Verification items for the finished model (mm, model axes). Round coordinates to 2 decimals unless told otherwise and drop trailing zeros. Order: outer loops, then holes, each group sorted by start corner. A loop starts at its lowest first (then second) coordinate and runs counter-clockwise, first axis right, second up. Notation, with made-up numbers: (73, -32.5) -> (107, -32.5) arc R29 ccw to (107, 4.5) -> close; hole circle Ø7 at (18, 20). An arc over 180 degrees is marked (long way). Put each result on its own line as item: value.
```python
from build123d import *

# Parameters (mm, degrees)
SKETCH1_W           = 32.5
SKETCH1_H           = 14
BOSS_EXTRUDE1_DEPTH = 1.3
SKETCH2_R           = 0.2
SKETCH2_W           = 0.64
SKETCH2_H           = 0.64
CUT_EXTRUDE1_DEPTH  = 2.3
SKETCH3_R           = 1.5
CUT_EXTRUDE2_DEPTH  = 10


with BuildPart() as part:
    # Sketch1 → Boss-Extrude1 (new body)
    with BuildSketch(Plane(origin=(0, 0, 0), x_dir=(1, 0, 0), z_dir=(0, 1, 0))):
        Rectangle(SKETCH1_W, SKETCH1_H)
    extrude(amount=BOSS_EXTRUDE1_DEPTH)

    # Sketch2 → Cut-Extrude1 (cut, through all)
    with BuildSketch(Plane(origin=(0, 1.3, 0), x_dir=(1, 0, 0), z_dir=(0, 1, 0))):
        with Locations((14.52, -5)):
            Circle(SKETCH2_R)
        with Locations((11.98, -5)):
            Circle(SKETCH2_R)
        with Locations((11.98, 5)):
            Circle(SKETCH2_R)
        with Locations((14.52, 5)):
            Circle(SKETCH2_R)
        with Locations((-15.25, 3.81)):
            Rectangle(SKETCH2_W, SKETCH2_H)
        with Locations((-15.25, 1.27)):
            Rectangle(SKETCH2_W, SKETCH2_H)
        with Locations((-15.25, -1.27)):
            Rectangle(SKETCH2_W, SKETCH2_H)
        with Locations((-15.25, -3.81)):
            Rectangle(SKETCH2_W, SKETCH2_H)
    extrude(amount=-CUT_EXTRUDE1_DEPTH, mode=Mode.SUBTRACT)

    # Sketch3 → Cut-Extrude2 (cut)
    with BuildSketch(Plane(origin=(0, 1.3, 0), x_dir=(1, 0, 0), z_dir=(0, 1, 0))):
        with Locations((-8.75, 0)):
            Circle(SKETCH3_R)
    extrude(amount=-CUT_EXTRUDE2_DEPTH, mode=Mode.SUBTRACT)


solid = part.part
```
Item 1: Sectioned sample at C-C, the plane z = 0. Record the boundary of the cut face in (x, y), then the cut area to 4 significant figures.
Geometry check:
outline: (-16.25, 0) -> (-10.25, 0) -> (-10.25, 1.3) -> (-16.25, 1.3) -> close; (-7.25, 0) -> (16.25, 0) -> (16.25, 1.3) -> (-7.25, 1.3) -> close
area: 38.35 mm2
Item 2: Material ranges on line 1 along X through (y, z) = (1.15, 5); line 2 along Z through (x, y) = (11.98, 0.65); line 3 along X through (y, z) = (0.85, 0), recorded low to high.
Geometry check:
line 1: -16.25 to 11.78, 12.18 to 14.32, 14.72 to 16.25
line 2: -7 to -5.2, -4.8 to 4.8, 5.2 to 7
line 3: -16.25 to -10.25, -7.25 to 16.25
Item 3: Sectioned sample at A-A, the plane x = -8.75. Record the boundary of the cut face in (y, z).
Geometry check:
outline: (0, -7) -> (1.3, -7) -> (1.3, -1.5) -> (0, -1.5) -> close; (0, 1.5) -> (1.3, 1.5) -> (1.3, 7) -> (0, 7) -> close
Item 4: Depth check by flat-ended pin: pin 1 Ø2.5 at (x, z) = (-8.75, 0) entering from -Y. Enter the tip coordinate at first touch or a pass-through.
Geometry check:
pin 1: through
Item 5: Release check for a two-part mould opening along Z. For faces 1 (the face through (-10.25, 0.66, -0.07)), 2 (the face through (16.25, 1, 0)), 3 (the face through (0, 1, -7)) record: pulls with the +Z half, pulls with the -Z half, needs draft (parallel to the pull), parting line crosses it, or undercut.
Geometry check:
face 1: undercut
face 2: needs draft
face 3: pulls with the -Z half
Item 6: Sectioned sample at B-B, the plane y = 0.65. Give the number of separate pieces and of enclosed holes in the cut face, then the cut area to 3 significant figures.
Geometry check:
separate pieces: 1
enclosed holes: 9
area: 446 mm2
